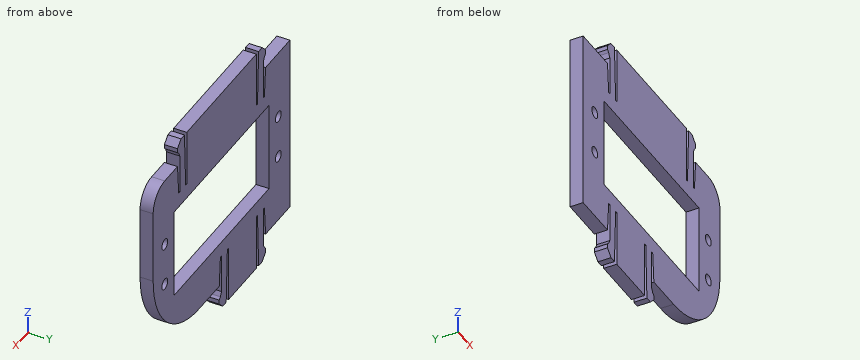
from build123d import *

# Parameters (mm, degrees)
BOSS_EXTRUDE4_DEPTH = 3
SKETCH7_R           = 1.25
SKETCH7_W           = 41
SKETCH7_H           = 21
CUT_EXTRUDE1_DEPTH  = 3
FILLET2_R           = 20
FILLET3_R           = 5


with BuildPart() as part:
    # Sketch1 → Boss-Extrude4 (new body)
    with BuildSketch(Plane(origin=(0, 0, 0), x_dir=(1, 0, 0), z_dir=(0, 1, 0))):
        Polygon((19, -21), (29.5, -21), (29.5, 21), (1, 21), (0.5, 13.997828908), (0, 13.997828908), (0, 22.997828908), (0.5, 23.997828908), (1, 24.497828908), (1, 25.497828908), (-0.5, 26.997828908), (-2, 26.997828908), (-2.5, 13.997828908), (-3, 13.997828908), (-3, 26.997828908), (-15, 26.997828908), (-15, 13.997828908), (-15.5, 13.997828908), (-16, 26.997828908), (-17.5, 26.997828908), (-19, 25.497828908), (-19, 24.497828908), (-18.5, 23.997828908), (-18, 22.997828908), (-18, 13.997828908), (-18.5, 13.997828908), (-19, 21), (-29.5, 21), (-29.5, -21), (-19, -21), (-18.5, -13.997828908), (-18, -13.997828908), (-18, -22.997828908), (-18.5, -23.997828908), (-19, -24.497828908), (-19, -25.497828908), (-17.5, -26.997828908), (-16, -26.997828908), (-15.5, -13.997828908), (-15, -13.997828908), (-15, -26.997828908), (15, -26.997828908), (15, -13.997828908), (15.5, -13.997828908), (16, -26.997828908), (17.5, -26.997828908), (19, -25.497828908), (19, -24.497828908), (18.5, -23.997828908), (18, -22.997828908), (18, -13.997828908), (18.5, -13.997828908), align=None)
    extrude(amount=BOSS_EXTRUDE4_DEPTH)

    # Sketch7 → Cut-Extrude1 (cut)
    with BuildSketch(Plane(origin=(0, 3, 0), x_dir=(1, 0, 0), z_dir=(0, 1, 0))):
        with Locations((-24.5, 5)):
            Circle(SKETCH7_R)
        with Locations((-24.5, -5)):
            Circle(SKETCH7_R)
        with Locations((24.5, -5)):
            Circle(SKETCH7_R)
        with Locations((24.5, 5)):
            Circle(SKETCH7_R)
        Rectangle(SKETCH7_W, SKETCH7_H)
    extrude(amount=-CUT_EXTRUDE1_DEPTH, mode=Mode.SUBTRACT)

    # Fillet2
    fillet2_edges = [part.edges().sort_by_distance(p)[0] for p in [
        (29.5, 1.5, -21),
    ]]
    fillet(fillet2_edges, radius=FILLET2_R)

    # Fillet3
    fillet3_edges = [part.edges().sort_by_distance(p)[0] for p in [
        (29.5, 1.5, 21),
    ]]
    fillet(fillet3_edges, radius=FILLET3_R)


solid = part.part
Work out the finished part from the listing and answer in its coordinate system (mm). Give positions to 0.01 mm unless a question says otherwise; leave off trailing zeros. Order: outer loops, then holes, each group sorted by start corner. A loop starts at its lowest first (then second) coordinate and runs counter-clockwise, first axis right, second up. Notation, with made-up numbers: (-4, 47.5) -> (22, 47.5) arc R22 ccw to (22, 76.5) -> close; hole circle Ø11 at (-39.75, -34.5). An arc over 180 degrees is marked (long way). Answer as a JSON object with one key per item and string values. Group by question number.
1. Flat-ended cylindrical pins translate along their axes: pin 1 Ø1.5 at (x, y) = (6, 2) entering from -Z; pin 2 Ø0.9 at (y, z) = (2, -23.5) entering from +X; pin 3 Ø0.6 at (x, y) = (0.5, 2) entering from -Z. Find the tip coordinate at first contact, or state that the pin passes through.
2. Section D-D on z = 17.5 is taken. Determine the outline of the cut face in (x, y).
3. Section A-A on x = -6 is taken. Determine the outline of the cut face in (y, z).
4. Consider line 1 along X through (y, z) = (0.7, 5); line 2 along Z through (x, y) = (-24.5, 2.3); line 3 along X through (y, z) = (0.8, -5). Determine where each line is inside the solid, lowest interval first. Write a range as [from, to].
5. Section C-C on x = -24.5 is taken. Determine the outline of the cut face in (y, z), plus the area to 3 significant figures.
6. Section B-B on z = -5 is taken. Determine the outline of the cut face in (x, y), plus the area to 3 significant figures.
Result sheet:
{
 "1": {"pin 1": "stops at z = -21", "pin 2": "stops at x = 0.48", "pin 3": "stops at z = -26.3"},
 "2": {"outline": "(-29.5, 0) -> (-18.75, 0) -> (-18.75, 3) -> (-29.5, 3) -> close; (-18, 0) -> (-15.63, 0) -> (-15.63, 3) -> (-18, 3) -> close; (-15, 0) -> (15, 0) -> (15, 3) -> (-15, 3) -> close; (15.63, 0) -> (18, 0) -> (18, 3) -> (15.63, 3) -> close; (18.75, 0) -> (29.27, 0) -> (29.27, 3) -> (18.75, 3) -> close"},
 "3": {"outline": "(0, -27) -> (3, -27) -> (3, -10.5) -> (0, -10.5) -> close; (0, 10.5) -> (3, 10.5) -> (3, 27) -> (0, 27) -> close"},
 "4": {"line 1": "x = [-29.5, -25.75], [-23.25, -20.5], [20.5, 23.25], [25.75, 29.5]", "line 2": "z = [-21, -6.25], [-3.75, 3.75], [6.25, 21]", "line 3": "x = [-29.5, -25.75], [-23.25, -20.5], [20.5, 23.25], [25.75, 29.1]"},
 "5": {"outline": "(0, -21) -> (3, -21) -> (3, -6.25) -> (0, -6.25) -> close; (0, -3.75) -> (3, -3.75) -> (3, 3.75) -> (0, 3.75) -> close; (0, 6.25) -> (3, 6.25) -> (3, 21) -> (0, 21) -> close", "area": "111 mm^2"},
 "6": {"outline": "(-29.5, 0) -> (-25.75, 0) -> (-25.75, 3) -> (-29.5, 3) -> close; (-23.25, 0) -> (-20.5, 0) -> (-20.5, 3) -> (-23.25, 3) -> close; (20.5, 0) -> (23.25, 0) -> (23.25, 3) -> (20.5, 3) -> close; (25.75, 0) -> (29.1, 0) -> (29.1, 3) -> (25.75, 3) -> close", "area": "37.8 mm^2"}
}
